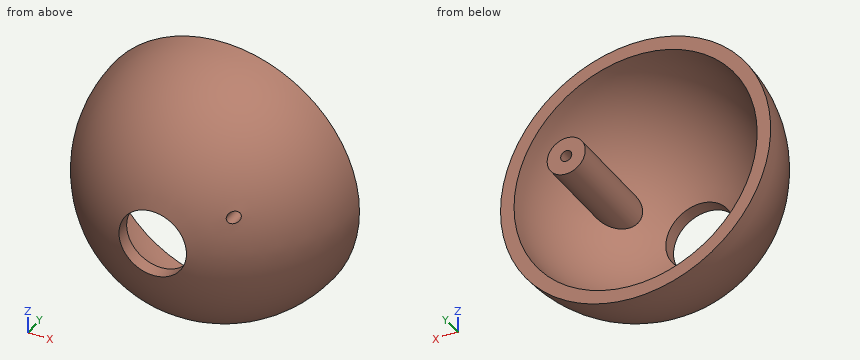
from build123d import *

# Parameters (mm, degrees)
F0_R     = 25.4
F0_R_2   = 1.0439291231
F1_DEPTH = 25.4
F3_T     = -2.54
F4_R     = 6.35
F5_DEPTH = 50.8


# Not quite as in the source:
# - a fillet or chamfer that OpenCascade refuses, or shapes differently, is made with other operations: its cross-section is extruded or revolved along the edge and cut away or added


with BuildPart() as f1:
    # F0 (on Front) → F1 (new body)
    with BuildSketch(Plane.XZ):
        Circle(F0_R)
        with Locations((13.0458941537, 7.0479529987)):
            Circle(F0_R_2, mode=Mode.SUBTRACT)
    extrude(amount=F1_DEPTH)

    # F2: fillet of radius 25.4 on 1 edges, made by hand

    # F2_s1 → F2_t2 (revolve, cut)
    with BuildSketch(Plane.XY):
        with BuildLine():
            ThreePointArc((25.4, 0), (17.9605122421, -17.9605122421), (0, -25.4))
            Line((0, -25.4), (25.4, -25.4))
            Line((25.4, -25.4), (25.4, 0))
        make_face()
    revolve(axis=Axis((0, -25.4, 0), (0, -1, 0)), mode=Mode.SUBTRACT)

    # F3
    f3_openings = [f1.faces().sort_by_distance(p)[0] for p in [
        (-0.022074, 0, -0.011925),
    ]]
    offset(amount=F3_T, openings=f3_openings)

    # F4 (on Front) → F5 (cut)
    with BuildSketch(Plane.XZ):
        Circle(F4_R)
    extrude(amount=F5_DEPTH, mode=Mode.SUBTRACT)


solid = f1.part
The model under review builds one solid part; all positions refer to its coordinate system, in mm. Coordinates: 2 decimals unless noted, no trailing zeros. Write each loop counter-clockwise with the first axis right and the second up, starting at its lowest first coordinate (ties: lowest second). Pieces come first, ordered by that corner, then holes. Notation, with made-up numbers: (2.25, -36.75) -> (6.25, -36.75) arc R17 ccw to (6.25, -32.75) -> close; hole circle Ø1 at (-5.5, 78.25). An arc over 180 degrees is marked (long way). Answer in a Markdown table with one row per item.
1. Clearance check with flat-ended pins moving along their axes: pin 1 Ø8 at (x, y) = (-10, -11) entering from -Z; pin 2 Ø1.5 at (y, z) = (-5.5, -11.5) entering from +X; pin 3 Ø12 at (x, z) = (-18, 0.5) entering from -Y; pin 4 Ø10 at (x, z) = (0, 0) entering from +Y. State where each tip first meets the part, or that it passes through.
Answers below:
| item | result |
|---|---|
| pin 1 | stops at z = -22.96 |
| pin 2 | stops at x = 22.39 |
| pin 3 | stops at y = -22.38 |
| pin 4 | passes through |
2. We need section D-D, the plane z = -19.5. State the section outline as (x, y) points, and give its area (3 significant figures).
Answers below:
| item | result |
|---|---|
| outline | (-16.28, 0) arc R16.28 ccw to (16.28, 0) -> (11.93, 0) arc R11.93 cw to (-11.93, 0) -> close |
| area | 193 mm^2 |
3. We need section B-B, the plane z = 0. State the section outline as (x, y) points, and give its area (3 significant figures).
Answers below:
| item | result |
|---|---|
| outline | (-25.4, 0) arc R25.4 ccw to (-6.35, -24.59) -> (-6.35, -21.96) arc R22.86 cw to (-22.86, 0) -> close; (6.35, -24.59) arc R25.4 ccw to (25.4, 0) -> (22.86, 0) arc R22.86 cw to (6.35, -21.96) -> close |
| area | 160 mm^2 |
4. Wall thickness on probe 1 along Z at (x, y) = (18, -11); probe 2 along X at (y, z) = (-15.25, 11.5); probe 3 along X at (y, z) = (-7.5, -6.5): over which ranges is each line inside the solid? List them lowest first. Write a range as [from, to].
Answers below:
| item | result |
|---|---|
| probe 1 | z = [-14.15, -8.81], [8.81, 14.15] |
| probe 2 | x = [-16.74, -12.56], [12.56, 16.74] |
| probe 3 | x = [-23.38, -20.59], [20.59, 23.38] |
5. We need section C-C, the plane y = -10.5. State the section outline as (x, z) points, and give its area (3 significant figures).
Answers below:
| item | result |
|---|---|
| outline | circle Ø46.26 at (0, 0); circle Ø7.17 at (13.05, 7.05); hole circle Ø40.61 at (0, 0); hole circle Ø2.09 at (13.05, 7.05) |
| area | 422 mm^2 |
6. We need section A-A, the plane x = 0. State the section outline as (y, z) points.
Answers below:
| item | result |
|---|---|
| outline | (-24.59, -6.35) arc R25.4 ccw to (0, -25.4) -> (0, -22.86) arc R22.86 cw to (-21.96, -6.35) -> close; (-24.59, 6.35) -> (-21.96, 6.35) arc R22.86 cw to (0, 22.86) -> (0, 25.4) arc R25.4 ccw to start |
